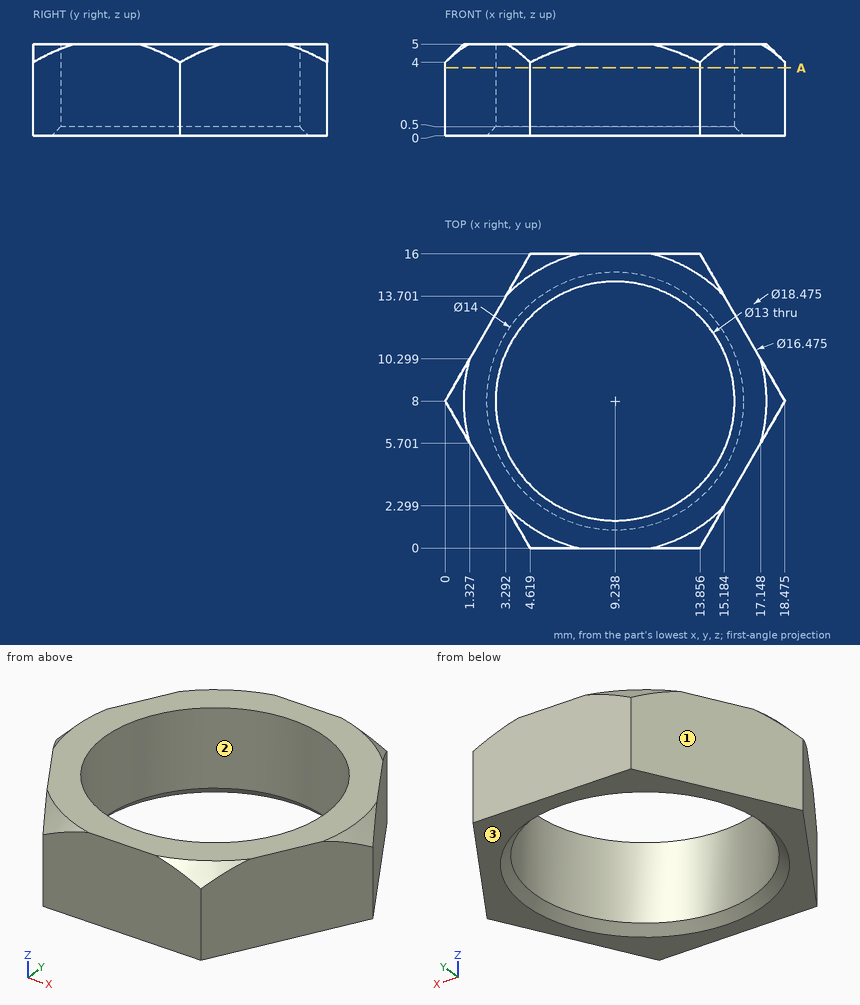
Part print with two shaded views. Sizes in mm from the minimum x, y, z corner. Coordinates: 2 decimals unless noted, no trailing zeros. Write each loop counter-clockwise with the first axis right and the second up, starting at its lowest first coordinate (ties: lowest second). Pieces come first, ordered by that corner, then holes.
1. Drill centre lines: probe 1 along Y at (x, z) = (9.5, 2.6) (1 decimal); probe 2 along Y at (x, z) = (12.25, 3.35); probe 3 along X at (y, z) = (2.75, 4.3) (1 decimal). Where is each one in solid material? Low to high.
Answer block:
probe 1: y = 0 to 1.5, 14.5 to 16
probe 2: y = 0 to 2.24, 13.76 to 16
probe 3: x = 3 to 5.4, 13.1 to 15.4
2. Drop flat-ended pins along their axis: pin 1 (3 mm diameter, centred on x = 16.5, z = 2, fed in from +Y); pin 2 (1 mm diameter, centred on y = 9.5, z = 2, fed in from +X). Give the stop position or say it passes through.
Answer block:
pin 1: stops at y = 14.02
pin 2: stops at x = 17.9
3. Band-saw the part on A-A, the plane z = 3.7. Give the cut face in (x, y) (1 decimal).
Answer block:
outline: (0, 8) - (4.6, 0) - (13.9, 0) - (18.5, 8) - (13.9, 16) - (4.6, 16) - close; hole circle Ø13 at (9.2, 8)
4. Pull direction X, two halves, no side cores. Call the marked faces 1, 2 and 3: released by +X, released by -X, zero draft, split by the parting line, or undercut.
Answer block:
face 1: released by -X
face 2: undercut
face 3: zero draft
